Build history of the part. All positions in model axes, mm. Face numbers are marked on the shaded views. Give positions to 0.01 mm unless a question says otherwise; leave off trailing zeros. Order: outer loops, then holes, each group sorted by start corner. A loop starts at its lowest first (then second) coordinate and runs counter-clockwise, first axis right, second up. Notation, with made-up numbers: (-15.75, 81) - (18.25, 81) arc R21 cw to (18.25, 119) - close; hole circle Ø1 at (57, -18.75). An arc over 180 degrees is marked (long way). Answer in a Markdown table with one row per item.
```python
from build123d import *

# Parameters (mm, degrees)
CYLINDER030_R          = 1.6
CYLINDER030_DEPTH      = 12
CYLINDER018_R          = 1.6
CYLINDER018_DEPTH      = 12
PRISM001_DEPTH         = 3
BOX021_W               = 8.5
BOX021_H               = 11
BOX021_DEPTH           = 7
CYLINDER029_R          = 1.6
CYLINDER029_DEPTH      = 10
CYLINDER029_ROLL_ANGLE = 90
CYLINDER016_R          = 1.6
CYLINDER016_DEPTH      = 10
CYLINDER016_ROLL_ANGLE = 90
BOX004_W               = 108
BOX004_H               = 3
BOX004_DEPTH           = 30
CYLINDER014_R          = 1.6
CYLINDER014_DEPTH      = 16
CYLINDER014_ROLL_ANGLE = 90
PRISM_DEPTH            = 3
BOX020_W               = 10
BOX020_H               = 11
BOX020_DEPTH           = 7
CHAMFER004_SIZE        = 1


with BuildPart() as cylinder030:
    # Cylinder030 → Cylinder030 (new body)
    with BuildSketch(Plane(origin=(3.6, 5.69, -7), x_dir=(1, 0, 0), z_dir=(0, 0, 1))):
        Circle(CYLINDER030_R)
    extrude(amount=CYLINDER030_DEPTH)


with BuildPart() as cylinder018:
    # Cylinder018 → Cylinder018 (new body)
    with BuildSketch(Plane(origin=(3.6, 5.69, -7), x_dir=(1, 0, 0), z_dir=(0, 0, 1))):
        Circle(CYLINDER018_R)
    extrude(amount=CYLINDER018_DEPTH)


with BuildPart() as prism001:
    # Prism001 → Prism001 (new body)
    with BuildSketch(Plane(origin=(3.6, 5.69, -7), x_dir=(1, 0, 0), z_dir=(0, 0, 1))):
        Polygon((3, 0), (1.5, 2.598076), (-1.5, 2.598076), (-3, 0), (-1.5, -2.598076), (1.5, -2.598076), align=None)
    extrude(amount=PRISM001_DEPTH)


with BuildPart() as cut008:
    # Box021 → Box021 (new body)
    with BuildSketch(Plane(origin=(-1.25, 0, -7), x_dir=(1, 0, 0), z_dir=(0, 0, 1))):
        with Locations((4.25, 5.5)):
            Rectangle(BOX021_W, BOX021_H)
    extrude(amount=BOX021_DEPTH)

    # Cut007: cut Prism001
    add(prism001.part, mode=Mode.SUBTRACT)


with BuildPart() as cut008_1:
    # Cut007 placement: moved
    add(cut008.part.moved(Location((0, 0, -1))))

    # Cut008: cut Cylinder018
    add(cylinder018.part, mode=Mode.SUBTRACT)


with BuildPart() as cut008_2:
    # Cut008 placement: moved
    add(cut008_1.part.moved(Location((92.5, 0, 0))))


with BuildPart() as cylinder029:
    # Cylinder029 → Cylinder029 (new body)
    with BuildSketch(Plane.XY):
        Circle(CYLINDER029_R)
    extrude(amount=CYLINDER029_DEPTH)


with BuildPart() as cylinder029_1:
    # Cylinder029 roll: moved
    add(cylinder029.part.rotate(Axis((0, 0, 0), (1, 0, 0)), CYLINDER029_ROLL_ANGLE))


with BuildPart() as cylinder029_2:
    # Cylinder029 placement: moved
    add(cylinder029_1.part.moved(Location((3.6, 5.69, -20.3))))


with BuildPart() as fusion010:
    # Cylinder016 → Cylinder016 (new body)
    with BuildSketch(Plane.XY):
        Circle(CYLINDER016_R)
    extrude(amount=CYLINDER016_DEPTH)


with BuildPart() as fusion010_1:
    # Cylinder016 roll: moved
    add(fusion010.part.rotate(Axis((0, 0, 0), (1, 0, 0)), CYLINDER016_ROLL_ANGLE))


with BuildPart() as fusion010_2:
    # Cylinder016 placement: moved
    add(fusion010_1.part.moved(Location((96, 5.69, -18.4))))

    # Fusion010: union Cylinder029
    add(cylinder029_2.part)


with BuildPart() as right_with_holes:
    # Box004 → Box004 (new body)
    with BuildSketch(Plane(origin=(-5, -3, -25), x_dir=(1, 0, 0), z_dir=(0, 0, 1))):
        with Locations((54, 1.5)):
            Rectangle(BOX004_W, BOX004_H)
    extrude(amount=BOX004_DEPTH)

    # Cut028: cut Fusion010
    add(fusion010_2.part, mode=Mode.SUBTRACT)


with BuildPart() as cylinder014:
    # Cylinder014 → Cylinder014 (new body)
    with BuildSketch(Plane.XY):
        Circle(CYLINDER014_R)
    extrude(amount=CYLINDER014_DEPTH)


with BuildPart() as cylinder014_1:
    # Cylinder014 roll: moved
    add(cylinder014.part.rotate(Axis((0, 0, 0), (1, 0, 0)), CYLINDER014_ROLL_ANGLE))


with BuildPart() as cylinder014_2:
    # Cylinder014 placement: moved
    add(cylinder014_1.part.moved(Location((3.6, 5.69, -20.3))))


with BuildPart() as prism:
    # Prism → Prism (new body)
    with BuildSketch(Plane(origin=(3.6, 5.69, -7), x_dir=(1, 0, 0), z_dir=(0, 0, 1))):
        Polygon((3, 0), (1.5, 2.598076), (-1.5, 2.598076), (-3, 0), (-1.5, -2.598076), (1.5, -2.598076), align=None)
    extrude(amount=PRISM_DEPTH)


with BuildPart() as right_side_final:
    # Box020 → Box020 (new body)
    with BuildSketch(Plane(origin=(-1.25, 0, -7), x_dir=(1, 0, 0), z_dir=(0, 0, 1))):
        with Locations((5, 5.5)):
            Rectangle(BOX020_W, BOX020_H)
    extrude(amount=BOX020_DEPTH)

    # Cut005: cut Prism
    add(prism.part, mode=Mode.SUBTRACT)


with BuildPart() as right_side_final_1:
    # Cut005 placement: moved
    add(right_side_final.part.moved(Location((0, 0, -1))))

    # Cut006: cut Cylinder014
    add(cylinder014_2.part, mode=Mode.SUBTRACT)

    # Fusion011: union Cut008, right with holes
    add(cut008_2.part)
    add(right_with_holes.part)

    # Chamfer004
    chamfer004_edges = [right_side_final_1.edges().sort_by_distance(p)[0] for p in [
        (95.5, 0, -8),
        (91.25, 0, -4.5),
        (8.75, 0, -4.5),
        (3.75, 0, -8),
    ]]
    chamfer(chamfer004_edges, length=CHAMFER004_SIZE)

    # Cut029: cut Cylinder030
    add(cylinder030.part, mode=Mode.SUBTRACT)


solid = right_side_final_1.part
```
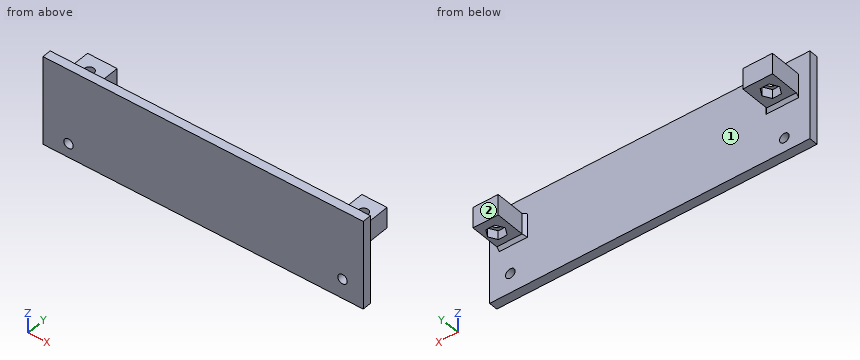
1. Cut at A-A on x = 3.6. Write the cut outline in (y, z), and give its area (3 significant figures).
Check result:
| item | result |
|---|---|
| outline | (-3, -25) - (0, -25) - (0, -21.9) - (-3, -21.9) - close; (-3, -18.7) - (0, -18.7) - (0, -9) - (1, -8) - (3.09, -8) - (3.09, -5) - (4.09, -5) - (4.09, -1) - (0, -1) - (0, 5) - (-3, 5) - close; (7.29, -5) - (8.29, -5) - (8.29, -8) - (11, -8) - (11, -1) - (7.29, -1) - close |
| area | 130 mm² |
2. Probe line 1 (X direction, y = 5.69, z = -4.2); line 2 (Y direction, x = 3.6, z = -2.15); line 3 (X direction, y = 8.75, z = -2.75). List the from-to ranges inside material, lowest first.
Check result:
| item | result |
|---|---|
| line 1 | x = -1.25 to 2, 5.2 to 8.75, 91.25 to 94.5, 97.7 to 99.75 |
| line 2 | y = -3 to 4.09, 7.29 to 11 |
| line 3 | x = -1.25 to 8.75, 91.25 to 99.75 |
3. Cut at D-D on x = 16. Write the cut outline in (y, z).
Check result:
| item | result |
|---|---|
| outline | (-3, -25) - (0, -25) - (0, 5) - (-3, 5) - close |
4. Drop flat-ended pins along their axis: P1, Ø4, axis at y = 5, z = -6.5, coming from the +X side; P2, Ø6, axis at y = 3.5, z = -1.5, coming from the -X side; P3, Ø3.5, axis at x = 96.1, y = 5.69, coming from the -Z side. Give the stop position or say it passes through.
Check result:
| item | result |
|---|---|
| P1 | stops at x = 99.75 |
| P2 | stops at x = -1.25 |
| P3 | stops at z = -5 |
5. Cut at B-B on z = -2.5. Write the cut outline in (x, y).
Check result:
| item | result |
|---|---|
| outline | (-5, -3) - (103, -3) - (103, 0) - (99.75, 0) - (99.75, 11) - (91.25, 11) - (91.25, 1) - (90.25, 0) - (9.75, 0) - (8.75, 1) - (8.75, 11) - (-1.25, 11) - (-1.25, 0) - (-5, 0) - close; hole circle Ø3.2 at (3.6, 5.69); hole circle Ø3.2 at (96.1, 5.69) |
6. Cut at C-C on x = 96.1. Write the cut outline in (y, z), and give its area (3 significant figures).
Check result:
| item | result |
|---|---|
| outline | (-3, -25) - (0, -25) - (0, -20) - (-3, -20) - close; (-3, -16.8) - (0, -16.8) - (0, -9) - (1, -8) - (3.09, -8) - (3.09, -5) - (4.09, -5) - (4.09, -1) - (0, -1) - (0, 5) - (-3, 5) - close; (7.29, -5) - (8.29, -5) - (8.29, -8) - (11, -8) - (11, -1) - (7.29, -1) - close |
| area | 130 mm² |
7. Two-plate mould, pull along X, no slides. Class the marked faces 1 and 2: +X half, -X half, draft (parallel to the pull), parting line (faces both ways), or undercut.
Check result:
| item | result |
|---|---|
| face 1 | undercut |
| face 2 | draft |
